Drawing for the job (mm, zero at the part's lowest x, y, z). Give positions to 0.01 mm unless a question says otherwise; leave off trailing zeros. Loops run counter-clockwise (first coordinate to the right, second up) from the corner with the lowest first, then second, coordinate; pieces in that order, holes last. Notation, with made-up numbers: M 71,47.25 L 81,47.25 A9 ccw 81,62.25 Z; hole C -27.75,-28.75 d3. An arc over 180 degrees is marked long. Answer in a Markdown table with one row per item. Add a question column.
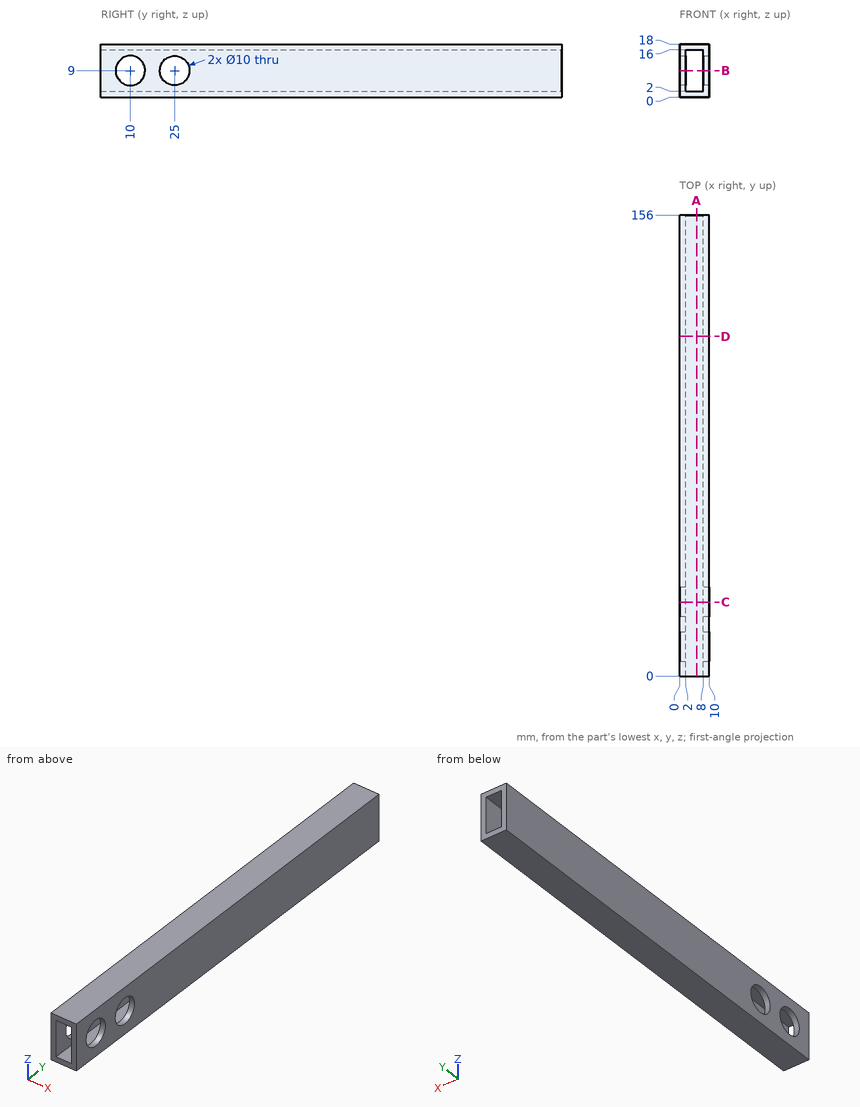
(1) Pin check, flat tip, straight feed: pin 1 (3 mm diameter, centred on x = 7, y = 45.5, fed in from -Z). Stop position of the tip, or through.
(2) Slice it at A-A, the plane x = 5.75. Give the cut face in (y, z).
(3) Wall check: line 1 (Y direction, x = 1.55, z = 9); line 2 (X direction, y = 117.5, z = 4.5); line 3 (Z direction, x = 4.5, y = 92). Give the ranges that are in metal, low to high.
(4) Slice it at C-C, the plane y = 25. Give the cut face in (x, z).
(5) Slice it at D-D, the plane y = 115. Give the cut face in (x, z).
(6) Slice it at B-B, the plane z = 9. Give the cut face in (x, y), then the cut area to 3 significant figures.
Solution:
| question | item | result |
|---|---|---|
| 1 | pin 1 | z = 0 |
| 2 | outline | M 0,0 L 156,0 L 156,2 L 0,2 Z; M 0,16 L 156,16 L 156,18 L 0,18 Z |
| 3 | line 1 | 0 to 5, 15 to 20, 30 to 156 |
| 3 | line 2 | 0 to 2, 8 to 10 |
| 3 | line 3 | 0 to 2, 16 to 18 |
| 4 | outline | M 0,0 L 10,0 L 10,4 L 8,4 L 8,2 L 2,2 L 2,4 L 0,4 Z; M 0,14 L 2,14 L 2,16 L 8,16 L 8,14 L 10,14 L 10,18 L 0,18 Z |
| 5 | outline | M 0,0 L 10,0 L 10,18 L 0,18 Z; hole M 2,2 L 8,2 L 8,16 L 2,16 Z |
| 6 | outline | M 0,0 L 2,0 L 2,5 L 0,5 Z; M 0,15 L 2,15 L 2,20 L 0,20 Z; M 0,30 L 2,30 L 2,156 L 0,156 Z; M 8,0 L 10,0 L 10,5 L 8,5 Z; M 8,15 L 10,15 L 10,20 L 8,20 Z; M 8,30 L 10,30 L 10,156 L 8,156 Z |
| 6 | area | 544 mm^2 |
